```python
from build123d import *

# Parameters (mm, degrees)
RESSALTO_EXTRUS_O1_DEPTH = 5


with BuildPart() as part:
    # Varredura1: sweep along a path in Esboço1
    with BuildLine(Plane.XY) as varredura1_path:
        Line((0, 0), (-140.664241345, 0))
        ThreePointArc((-140.664241345, 0), (-154.486995682, -11.779310345), (-145.049390997, -27.295505351))
        Line((-145.049390997, -27.295505351), (126.870742838, -116.980737218))
        ThreePointArc((126.870742838, -116.980737218), (204.904617075, -69.517241379), (145.664241345, 0))
        Line((145.664241345, 0), (5, 0))
    # Esboço2 → Varredura1 (sweep)
    with BuildSketch(Plane(origin=(0, 0, 0), x_dir=(0, 0, -1), z_dir=(1, 0, 0))):
        Polygon((-8.4, 10), (8.4, 10), (5.720508076, 0), (-5.720508076, 0), align=None)
    sweep(path=varredura1_path.line)

    # Esboço3 → Ressalto-extrusão1 (add)
    with BuildSketch(Plane(origin=(0, 0, 0), x_dir=(0, 0, -1), z_dir=(1, 0, 0))):
        Polygon((-8.4, 10), (-5.720508076, 0), (5.720508076, 0), (8.4, 10), align=None)
    extrude(amount=RESSALTO_EXTRUS_O1_DEPTH)


solid = part.part
```
Here's how the part is built. I have some questions about the finished solid (model axes, mm). A direction names the side the tool comes from. Coordinates: 2 decimals unless noted, no trailing zeros. Order: outer loops, then holes, each group sorted by start corner. A loop starts at its lowest first (then second) coordinate and runs counter-clockwise, first axis right, second up. Notation, with made-up numbers: (-31, 16.25) - (9, 16.25) arc R23 cw to (9, 41.25) - close; hole circle Ø7 at (-37, 49). An arc over 180 degrees is marked (long way). One line per question, with ' | ' between items. Start each with the question number.
1. I'm going to push flat-ended pins straight in: pin 1 Ø4 at (y, z) = (-48.5, 3) entering from +X; pin 2 Ø10 at (x, z) = (105.5, 0) entering from -Y; pin 3 Ø5 at (x, y) = (99.5, -107.5) entering from -Z. Where does each tip first touch, or does it pass through?
2. Please list where these lines run through material, in increasing order: line 1 along Z through (x, y) = (62.5, -106); line 2 along Y through (x, z) = (-124, -2.75); line 3 along Y through (x, z) = (-92.5, -4). Write a range as [from, to].
3. If we section it at B-B (x = 52): Write out the boundary of the cut face in (y, z), and give its area (3 significant figures).
4. If we section it at A-A (z = 1): Write out the boundary of the cut face in (x, y), and give its area (3 significant figures).
5. Which directions (+Z, -Z, +X, -X, +Y, -Y) give clear straight access to the entire face, cutting with the end or side of a thin tool? Please do faces 1 (the conical face through (-154.92, -11.42, 5.85)), 2 (the flat face through (0, 0, 0)), 3 (the flat face through (0.5, 4.93, -7.04)).
6. If we section it at C-C (y = -60): Write out the boundary of the cut face in (x, z).
Model answer:
1) pin 1: stops at x = 215.02 | pin 2: stops at y = -122.11 | pin 3: stops at z = -6.28
2) line 1: z = [-8.33, 8.33] | line 2: y = [-44.77, -34.24], [0, 10] | line 3: y = [-55.16, -44.63], [0, 10]
3) outline: (-102.82, -8.4) - (-92.29, -5.72) - (-92.29, 5.72) - (-102.82, 8.4) - close; (0, -5.72) - (10, -8.4) - (10, 8.4) - (0, 5.72) - close | area: 290 mm²
4) outline: (-148.18, -36.79) - (123.74, -126.48) arc R70 ccw (long way) to (145.66, 10) - (-140.66, 10) arc R24 ccw to start; hole (-145.05, -27.3) - (126.87, -116.98) arc R60 ccw (long way) to (145.66, 0) - (-140.66, 0) arc R14 ccw to start | area: 8,510 mm²
5) face 1: +Z | face 2: +Z, -Z | face 3: -Z
6) outline: (-77.82, -8.4) - (-45.89, -5.72) - (-45.89, 5.72) - (-77.82, 8.4) - close; (205.66, -5.72) - (215.66, -8.4) - (215.66, 8.4) - (205.66, 5.72) - close
